For this review, take the finished solid that the model builds, in its own axes (mm). A direction names the side the tool comes from. Give positions to 0.01 mm unless a question says otherwise; leave off trailing zeros. Write each loop counter-clockwise with the first axis right and the second up, starting at its lowest first coordinate (ties: lowest second). Pieces come first, ordered by that corner, then holes. Notation, with made-up numbers: M -13.5,21.25 L 16.5,21.25 A8 cw 16.5,29.25 Z; hole C 6,83.25 d9. An arc over 180 degrees is marked long. Write item = value, one per line.
```python
from build123d import *

# Parameters (mm, degrees)
SKETCH1_W            = 35.999968648
SKETCH1_H            = 39.60056603
BOSS_EXTRUDE1_DEPTH  = 33.93
SKETCH2_W            = 28.93
SKETCH2_H            = 5
CUT_EXTRUDE1_DEPTH   = 64.367558518
SKETCH3_W            = 16
SKETCH3_H            = 5
CUT_EXTRUDE2_DEPTH   = 64.367558518
CUT_EXTRUDE3_DEPTH   = 61.369212453
SKETCH5_W            = 30.4
SKETCH5_H            = 7.2
CUT_EXTRUDE4_DEPTH   = 31.93
CUT_EXTRUDE5_DEPTH   = 63.319559309
BOSS_EXTRUDE2_REACH  = 65.368
BOSS_EXTRUDE3_DEPTH  = 5
SKETCH16_W           = 35.999968648
SKETCH16_H           = 10
BOSS_EXTRUDE8_DEPTH  = 3
SKETCH12_W           = 35.999968648
SKETCH12_H           = 45.60056603
CUT_EXTRUDE6_DEPTH   = 2
FILLET1_R            = 1.5875
MOVE_START           = -34.93
MOVE_FACE1_OUTLINE_W = 35.999968648
MOVE_FACE1_OUTLINE_H = 29.60056603
MOVE_FACE1_DEPTH     = 1


# Read off the part's stored shape, not the designer's step: Move Face1
with BuildPart() as part:
    # Sketch1 → Boss-Extrude1 (new body)
    with BuildSketch(Plane.XY):
        with Locations((17.999984324, 19.800283015)):
            Rectangle(SKETCH1_W, SKETCH1_H)
    extrude(amount=-BOSS_EXTRUDE1_DEPTH)

    # Sketch2 → Cut-Extrude1 (cut, through all)
    with BuildSketch(Plane(origin=(35.999968648, 0, 0), x_dir=(0, 0, -1), z_dir=(1, 0, 0))):
        with Locations((19.465, 37.10056603)):
            Rectangle(SKETCH2_W, SKETCH2_H)
        with Locations((19.465, 2.5)):
            Rectangle(SKETCH2_W, SKETCH2_H)
    extrude(amount=-CUT_EXTRUDE1_DEPTH, mode=Mode.SUBTRACT)

    # Sketch3 → Cut-Extrude2 (cut, through all)
    with BuildSketch(Plane.XY):
        with Locations((17.999984324, 37.10056603)):
            Rectangle(SKETCH3_W, SKETCH3_H)
        with Locations((17.999984324, 2.5)):
            Rectangle(SKETCH3_W, SKETCH3_H)
    extrude(amount=-CUT_EXTRUDE2_DEPTH, mode=Mode.SUBTRACT)

    # Sketch4 → Cut-Extrude3 (cut, through all)
    with BuildSketch(Plane(origin=(0, 34.60056603, 0), x_dir=(1, 0, 0), z_dir=(0, 1, 0))):
        Polygon((9.999984324, 0), (17.999984324, 5), (25.999984324, 0), align=None)
    extrude(amount=-CUT_EXTRUDE3_DEPTH, mode=Mode.SUBTRACT)

    # Sketch5 → Cut-Extrude4 (cut)
    with BuildSketch(Plane.XY):
        with Locations((17.999984324, 11.4)):
            Rectangle(SKETCH5_W, SKETCH5_H)
        with Locations((17.999984324, 28.20056603)):
            Rectangle(SKETCH5_W, SKETCH5_H)
    extrude(amount=-CUT_EXTRUDE4_DEPTH, mode=Mode.SUBTRACT)

    # Sketch6 → Cut-Extrude5 (cut, through all)
    with BuildSketch(Plane.XY.offset(-31.93)):
        with BuildLine():
            Line((15.109984324, 29.66056603), (20.889984324, 29.66056603))
            ThreePointArc((20.889984324, 29.66056603), (22.469984324, 28.08056603), (20.889984324, 26.50056603))
            Line((20.889984324, 26.50056603), (15.109984324, 26.50056603))
            ThreePointArc((15.109984324, 26.50056603), (13.529984324, 28.08056603), (15.109984324, 29.66056603))
        make_face()
        with BuildLine():
            Line((15.109984324, 12.86), (20.889984324, 12.86))
            ThreePointArc((20.889984324, 12.86), (22.469984324, 11.28), (20.889984324, 9.7))
            Line((20.889984324, 9.7), (15.109984324, 9.7))
            ThreePointArc((15.109984324, 9.7), (13.529984324, 11.28), (15.109984324, 12.86))
        make_face()
    extrude(amount=-CUT_EXTRUDE5_DEPTH, mode=Mode.SUBTRACT)

    # Sketch7 → Boss-Extrude2 (add, up to next)
    with BuildSketch(Plane.XY, mode=Mode.PRIVATE) as boss_extrude2_sk1:
        Polygon((2.799984324, 28.422935376), (2.799984324, 27.45056603), (3.299984324, 27.45056603), (3.299984324, 27.896781183), align=None)
    boss_extrude2_tool1 = extrude(boss_extrude2_sk1.sketch, amount=-BOSS_EXTRUDE2_REACH, mode=Mode.PRIVATE) - part.part
    # Sketch7 → Boss-Extrude2 (add, up to next)
    with BuildSketch(Plane.XY, mode=Mode.PRIVATE) as boss_extrude2_sk2:
        Polygon((2.799984324, 11.622369346), (2.799984324, 10.65), (3.299984324, 10.65), (3.299984324, 11.096215154), align=None)
    boss_extrude2_tool2 = extrude(boss_extrude2_sk2.sketch, amount=-BOSS_EXTRUDE2_REACH, mode=Mode.PRIVATE) - part.part
    boss_extrude2_1 = boss_extrude2_tool1.solids().sort_by_distance((3.019076, 27.821475, 0))[0]
    add(boss_extrude2_1)
    boss_extrude2_2 = boss_extrude2_tool2.solids().sort_by_distance((3.019076, 11.020909, 0))[0]
    add(boss_extrude2_2)
    boss_extrude2 = boss_extrude2_1 + boss_extrude2_2  # Boss-Extrude2 as one shape, for the pattern or mirror that repeats it

    # Mirror1: Boss-Extrude2 across plane
    add(boss_extrude2.mirror(Plane(origin=(17.999984324, 0, 0), x_dir=(0, 0, 1), z_dir=(1, 0, 0))))

    # Sketch8 → Boss-Extrude3 (add)
    with BuildSketch(Plane(origin=(0, 34.60056603, 0), x_dir=(1, 0, 0), z_dir=(0, 1, 0))):
        Polygon((9.999984324, 0), (17.999984324, 5), (25.999984324, 0), (35.999968648, 0), (35.999968648, 10), (0, 10), (0, 0), align=None)
    boss_extrude3 = extrude(amount=BOSS_EXTRUDE3_DEPTH)

    # Sketch16 → Boss-Extrude8 (add)
    with BuildSketch(Plane(origin=(0, 39.60056603, 0), x_dir=(1, 0, 0), z_dir=(0, 1, 0))):
        with Locations((17.999984324, 5)):
            Rectangle(SKETCH16_W, SKETCH16_H)
    boss_extrude8 = extrude(amount=BOSS_EXTRUDE8_DEPTH)

    # Mirror2: Boss-Extrude3, Boss-Extrude8 across plane
    add(boss_extrude3.mirror(Plane.ZX.offset(19.800283015)))
    add(boss_extrude8.mirror(Plane.ZX.offset(19.800283015)))

    # Sketch12 → Cut-Extrude6 (cut)
    with BuildSketch(Plane.XY):
        with Locations((17.999984324, 19.800283015)):
            Rectangle(SKETCH12_W, SKETCH12_H)
        Polygon((2.799984324, 39.600283015), (33.199984324, 39.600283015), (33.199984324, 28.422935376), (32.699984324, 27.896781183), (32.699984324, 27.45056603), (33.199984324, 27.45056603), (33.199984324, 11.622369346), (32.699984324, 11.096215154), (32.699984324, 10.65), (33.199984324, 10.65), (33.199984324, 0.000283015), (2.799984324, 0.000283015), (2.799984324, 10.65), (3.299984324, 10.65), (3.299984324, 11.096215154), (2.799984324, 11.622369346), (2.799984324, 27.45056603), (3.299984324, 27.45056603), (3.299984324, 27.896781183), (2.799984324, 28.422935376), align=None, mode=Mode.SUBTRACT)
    extrude(amount=-CUT_EXTRUDE6_DEPTH, mode=Mode.SUBTRACT)

    # Fillet1
    fillet1_edges = [part.edges().sort_by_distance(p)[0] for p in [
        (33.199984324, 39.600283015, -1),
        (2.799984324, 0.000283015, -1),
        (2.799984324, 39.600283015, -1),
        (33.199984324, 0.000283015, -1),
    ]]
    fillet(fillet1_edges, radius=FILLET1_R)

    # Move Face1 outline → Move Face1 (add)
    with BuildSketch(Plane.XY.offset(MOVE_START)):
        with Locations((17.999984324, 19.800283015)):
            Rectangle(MOVE_FACE1_OUTLINE_W, MOVE_FACE1_OUTLINE_H)
        with BuildLine():
            ThreePointArc((15.109984324, 9.7), (13.529984324, 11.28), (15.109984324, 12.86))
            Line((15.109984324, 12.86), (20.889984324, 12.86))
            ThreePointArc((20.889984324, 12.86), (22.469984324, 11.28), (20.889984324, 9.7))
            Line((20.889984324, 9.7), (15.109984324, 9.7))
        make_face(mode=Mode.SUBTRACT)
        with BuildLine():
            ThreePointArc((15.109984324, 26.50056603), (13.529984324, 28.08056603), (15.109984324, 29.66056603))
            Line((15.109984324, 29.66056603), (20.889984324, 29.66056603))
            ThreePointArc((20.889984324, 29.66056603), (22.469984324, 28.08056603), (20.889984324, 26.50056603))
            Line((20.889984324, 26.50056603), (15.109984324, 26.50056603))
        make_face(mode=Mode.SUBTRACT)
    extrude(amount=MOVE_FACE1_DEPTH)


solid = part.part
```
1. We need section A-A, the plane z = -7. Write out the cut boundary in (x, y).
Responses:
outline = M 0,-3 L 36,-3 L 36,42.6 L 0,42.6 Z; hole M 2.8,7.8 L 33.2,7.8 L 33.2,10.65 L 32.7,10.65 L 32.7,11.1 L 33.2,11.62 L 33.2,15 L 2.8,15 L 2.8,11.62 L 3.3,11.1 L 3.3,10.65 L 2.8,10.65 Z; hole M 2.8,24.6 L 33.2,24.6 L 33.2,27.45 L 32.7,27.45 L 32.7,27.9 L 33.2,28.42 L 33.2,31.8 L 2.8,31.8 L 2.8,28.42 L 3.3,27.9 L 3.3,27.45 L 2.8,27.45 Z
2. The part is to be moulded in two halves that separate along X. For faces 1 (the face through (2.8, 13, -17)), 2 (the face through (3.28, 39.15, -1.01)), 3 (the face through (32.72, 0.45, -1.01)), 4 (the face through (18, 1, -10)), say which applies: +X half, -X half, draft (parallel to the pull), parting line (faces both ways), or undercut.
Responses:
face_1 = undercut
face_2 = -X half
face_3 = +X half
face_4 = draft
3. We need section B-B, the plane x = 8. Write out the cut boundary in (y, z).
Responses:
outline = M -3,-10 L 5,-10 L 5,-34.93 L 34.6,-34.93 L 34.6,-10 L 42.6,-10 L 42.6,-2 L 39.6,-2 L 39.6,0 L 31.8,0 L 31.8,-31.93 L 24.6,-31.93 L 24.6,0 L 15,0 L 15,-31.93 L 7.8,-31.93 L 7.8,0 L 0,0 L 0,-2 L -3,-2 Z
4. We need section D-D, the plane x = 19. Write out the cut boundary in (y, z) (3 decimals).
Responses:
outline = M -3,-10 L 5,-10 L 5,-34.93 L 9.7,-34.93 L 9.7,-31.93 L 7.8,-31.93 L 7.8,-4.375 L 0,-4.375 L 0,-2 L -3,-2 Z; M 12.86,-34.93 L 26.501,-34.93 L 26.501,-31.93 L 24.601,-31.93 L 24.601,-4.375 L 15,-4.375 L 15,-31.93 L 12.86,-31.93 Z; M 29.661,-34.93 L 34.601,-34.93 L 34.601,-10 L 42.601,-10 L 42.601,-2 L 39.601,-2 L 39.601,-4.375 L 31.801,-4.375 L 31.801,-31.93 L 29.661,-31.93 Z
5. Insertion check: P1, Ø10, axis at x = 12.5, y = 36.5, coming from the -Z side; P2, Ø2, axis at x = 28.5, z = -0.5, coming from the -Y side; P3, Ø1.6, axis at y = 19, z = -0.5, coming from the -X side; P4, Ø12.5, axis at x = 20.5, z = -28.5, coming from the +Y side. Each pin has a flat end and moves straight along its axis. Give the tip position at first contact, or say it passes through.
Responses:
P1 = -34.93
P2 = 0
P3 = 2.8
P4 = 34.6
6. Machinability: for faces 5 (the face through (32.75, 39.12, -1.01)), 6 (the face through (18, 5, -23)), 7 (the face through (2.8, 35, -1)), 8 (the face through (8, 39.6, -1)), 9 (the face through (33.2, 9, -17)), which of the approach directions +Z, -Z, +X, -X, +Y, -Y give a long, thin tool a straight path to every point of the face, cutting with its end or side? Answer none if there is none.
Responses:
face_5 = +Z, +X, +Y
face_6 = -Z, +X, -X, -Y
face_7 = +Z, -X, +Y, -Y
face_8 = +Z, +X, -X, +Y
face_9 = +Z
7. For line 1 along Y through (x, z) = (21, -14); line 2 along Y through (x, z) = (4, -5); line 3 along X through (y, z) = (12, -21), list the stretches that pass through material, from the lowest coordinate up. Write a range as from..to.
Responses:
line_1 = 5..7.8, 15..24.6, 31.8..34.6
line_2 = -3..7.8, 15..24.6, 31.8..42.6
line_3 = 0..2.8, 33.2..36
8. We need section C-C, the plane y = 17. Write out the cut boundary in (x, z), then the cut area to 3 significant figures.
Responses:
outline = M 0,-34.93 L 36,-34.93 L 36,-2 L 33.2,-2 L 33.2,0 L 26,0 L 18,-5 L 10,0 L 2.8,0 L 2.8,-2 L 0,-2 Z
area = 1,210 mm2
